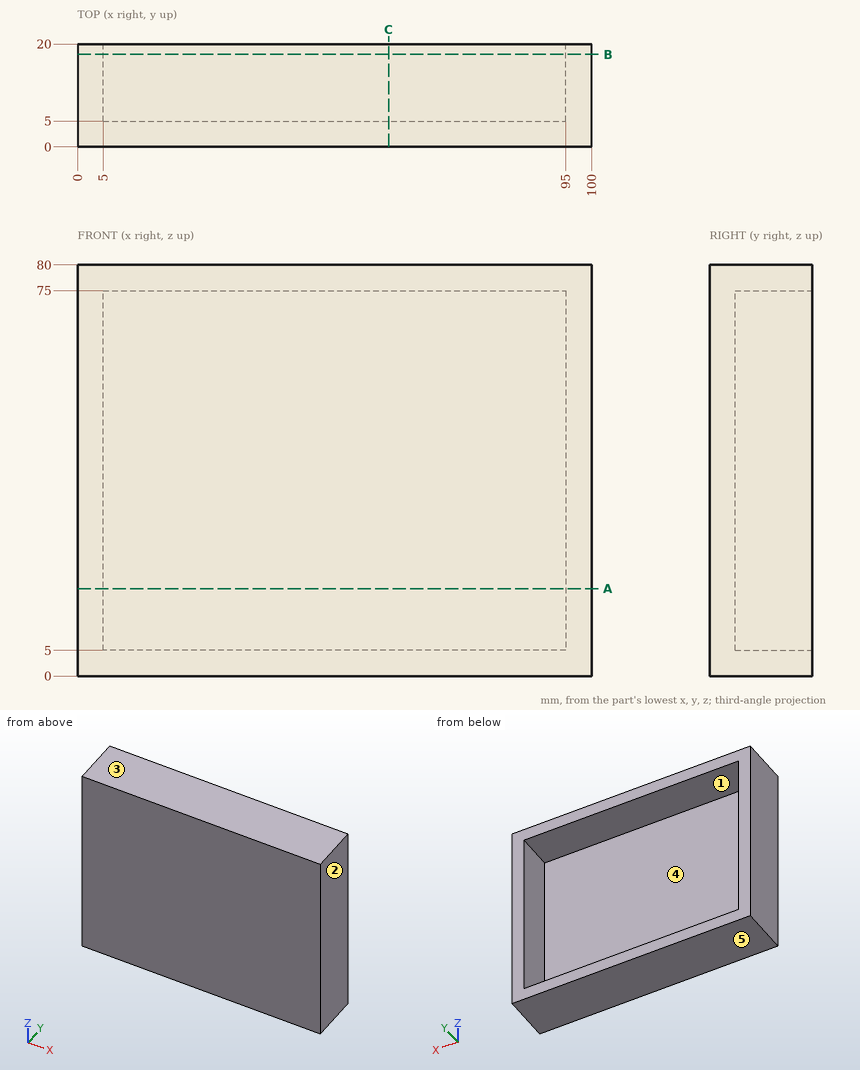
Check sheet for the drawn part. Datum: minimum x, y, z corner. Units: mm. A direction names the side the tool comes from. Round coordinates to 2 decimals unless told otherwise and drop trailing zeros. Loops run counter-clockwise (first coordinate to the right, second up) from the corner with the lowest first, then second, coordinate; pieces in that order, holes last. Notation, with made-up numbers: (-25.75, -12) - (-10.75, -12) arc R26 ccw to (-10.75, 19) - close; hole circle Ø7 at (24, 49). An arc over 180 degrees is marked (long way). Write item = value, one per line. Start each with the question number.
1. Mould release check, pull along X, two halves, no side actions. Record for the marked faces 1, 2 and 3: released by +X, released by -X, zero draft, split by the parting line, or undercut.
2. Thickness scan on line 1 (X direction, y = 6, z = 74.5); line 2 (Z direction, x = 88, y = 7.25); line 3 (Y direction, x = 75, z = 33). Record the ranges inside material, lowest first.
3. Section check A-A on z = 17. Enter the section's corners in (x, y).
4. Set-up check for the marked faces 4 and 5: record each of +Z, -Z, +X, -X, +Y, -Y from which the full face is reachable in a straight line by a thin tool's end or side.
5. Section check C-C on x = 60.5. Enter the section's corners in (y, z), then the cut area to 3 significant figures.
6. Section check B-B on y = 18. Enter the section's corners in (x, z), then the cut area to 3 significant figures.
Working result:
q1.face_1 = undercut
q1.face_2 = released by +X
q1.face_3 = zero draft
q2.line_1 = 0 to 5, 95 to 100
q2.line_2 = 0 to 5, 75 to 80
q2.line_3 = 0 to 5
q3.outline = (0, 0) - (100, 0) - (100, 20) - (95, 20) - (95, 5) - (5, 5) - (5, 20) - (0, 20) - close
q4.face_4 = +Y
q4.face_5 = -Z, +X, -X, +Y, -Y
q5.outline = (0, 0) - (20, 0) - (20, 5) - (5, 5) - (5, 75) - (20, 75) - (20, 80) - (0, 80) - close
q5.area = 550 mm^2
q6.outline = (0, 0) - (100, 0) - (100, 80) - (0, 80) - close; hole (5, 5) - (95, 5) - (95, 75) - (5, 75) - close
q6.area = 1,700 mm^2
